```python
from build123d import *

# Parameters (mm, degrees)
SWEEP_THIN1_PROFILE_R   = 30
SWEEP_THIN1_PROFILE_R_2 = 20
EXTRUDE_THIN1_START     = 20
EXTRUDE_THIN1_DEPTH     = 760


with BuildPart() as part:
    # Sweep-Thin1: sweep along a path in Sketch2
    with BuildLine(Plane(origin=(0, 0, 0), x_dir=(0, 0, -1), z_dir=(1, 0, 0))) as sweep_thin1_path:
        Line((0, 0), (120, 0))
        Line((120, 0), (226.066017178, -106.066017178))
        Line((226.066017178, -106.066017178), (419.251182436, -54.302208157))
    # Sweep-Thin1 profile (on start of the path) → Sweep-Thin1 (sweep)
    with BuildSketch(Plane(origin=(0, 0, 0), x_dir=(-1, 0, 0), z_dir=(0, 0, -1))):
        Circle(SWEEP_THIN1_PROFILE_R)
        Circle(SWEEP_THIN1_PROFILE_R_2, mode=Mode.SUBTRACT)
    sweep(path=sweep_thin1_path.line, transition=Transition.RIGHT)

    # Sketch13 → Extrude-Thin1 (add)
    with BuildSketch(Plane(origin=(0, 0, 0), x_dir=(0, 0, -1), z_dir=(1, 0, 0)).offset(EXTRUDE_THIN1_START)):
        Polygon((226.066017178, -106.066017178), (419.251182436, -54.302208157), (424.427563338, -73.620724683), (231.24239808, -125.384533704), align=None)
    extrude(amount=EXTRUDE_THIN1_DEPTH)

    # Mirror4: part across plane


with BuildPart() as part_1:
    add(part.part)
    add(part.part.mirror(Plane(origin=(405, 0, 0), x_dir=(0, 0, 1), z_dir=(1, 0, 0))))


solid = part_1.part
```
Part model, mm, in its own coordinate system. A direction names the side the tool comes from. Give positions to 0.01 mm unless a question says otherwise; leave off trailing zeros. Loops run counter-clockwise (first coordinate to the right, second up) from the corner with the lowest first, then second, coordinate; pieces in that order, holes last. Notation, with made-up numbers: M -19,-10.75 L 40,-10.75 A23 cw 40,3.25 Z; hole C 69,-16 d9. An arc over 180 degrees is marked long. Return JSON: item names as keys, results as strings.
1) Saw through at B-B, the plane x = 810. List the corners of the cut face in (y, z), then the cut area to 3 significant figures.
Calculated:
{"outline": "M -139.53,-217.1 L -83.28,-427.02 L -73.62,-424.43 L -128.37,-220.09 L -20,-111.72 L -20,0 L -30,0 L -30,-107.57 Z; M -83.76,-232.04 L -34.98,-414.07 L -25.32,-411.49 L -72.61,-235.03 L 30,-132.43 L 30,0 L 20,0 L 20,-128.28 Z", "area": "9,400 mm2"}
2) Saw through at D-D, the plane y = -117.5. Count the separate pieces of the cut face and the enclosed holes in it, then the cut area to 3 significant figures.
Calculated:
{"separate pieces": "1", "enclosed holes": "2", "area": "30,000 mm2"}
3) 3-axis set-ups, long thin cutter, end or side, ignore diameter. For faces 1 (the face through (3.905, 29.745, -67.14)), 2 (the face through (4.34, -100.15, -323.57)): which of +Z, -Z, +X, -X, +Y, -Y reach the whole face in a straight line?
Calculated:
{"face 1": "+Z", "face 2": "none"}
4) Drill centre lines: line 1 (Y direction, x = 0, z = -46.5); line 2 (X direction, y = -82.5, z = -258); line 3 (X direction, y = -60.5, z = -151.5). Where is each one in solid material? Low to high.
Calculated:
{"line 1": "y = -30 to -20, 20 to 30", "line 2": "x = -26.26 to -13.78, 13.78 to 26.26, 783.74 to 796.22, 823.78 to 836.26", "line 3": "x = -21.9 to 21.9, 788.1 to 831.9"}
5) Saw through at A-A, the plane z = -82. List the corners of the cut face in (x, y), then the cut area to 3 significant figures.
Calculated:
{"outline": "C 0,0 d60; C 810,0 d60; hole C 0,0 d40; hole C 810,0 d40", "area": "3,140 mm2"}
6) Saw through at C-C, the plane x = 160. List the corners of the cut face in (y, z).
Calculated:
{"outline": "M -125.38,-231.24 L -73.62,-424.43 L -54.3,-419.25 L -106.07,-226.07 Z"}
7) Pull direction Y, two halves, no side cores. Call faces 3 (the face through (410.36, -99.14, -329.19)), 4 (the face through (4.34, -68.83, -161.22)), 5 (the face through (399.75, -80.546, -321.306)): released by +Y, released by -Y, zero draft, split by the parting line, or undercut.
Calculated:
{"face 3": "released by -Y", "face 4": "undercut", "face 5": "released by +Y"}
8) Flat gauge pins, fed straight in: pin 1 Ø3 at (x, z) = (487, -239) entering from -Y; pin 2 Ø6 at (y, z) = (-74, -303.5) entering from +X; pin 3 Ø1.5 at (y, z) = (-35.5, -116) entering from -X. Where does each tip first touch, or does it go through?
Calculated:
{"pin 1": "stops at y = -123.71", "pin 2": "stops at x = 838.93", "pin 3": "stops at x = -12.7"}
